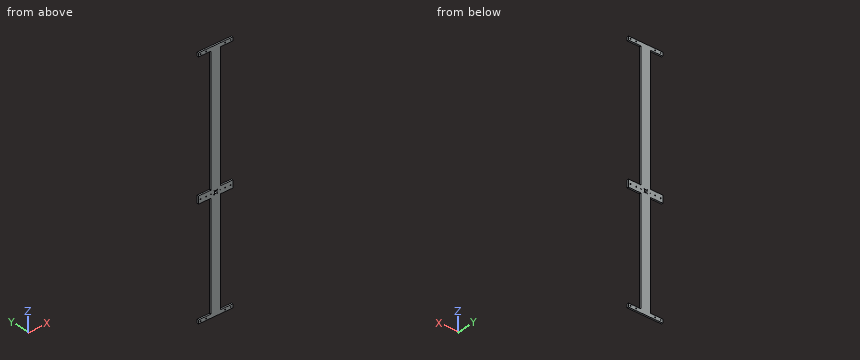
from build123d import *

# Parameters (mm, degrees)
SKETCH1_W                 = 108.8
SKETCH1_H                 = 23
MOUNT_BASE_DEPTH          = 5
SKETCH2_R                 = 1
SKETCH2_R_2               = 4.5
BRACKET_SCREW_HOLES_DEPTH = 5
SKETCH3_R                 = 1.5875
ANTENNA_SCREW_HOLES_DEPTH = 5
SKETCH6_W                 = 30
SKETCH6_H                 = 5
DIRECTOR_EXTENSION_DEPTH  = 328.35
SKETCH7_W                 = 108.8
SKETCH7_H                 = 5
DIRECTOR_MOUNT_DEPTH      = 11.5
SKETCH10_W                = 30
SKETCH10_H                = 5
REFLECTOR_EXTENSION_DEPTH = 394.02
SKETCH11_W                = 108.8
SKETCH11_H                = 5
REFLECTOR_MOUNT_DEPTH     = 11.5
LPATTERN1_COUNT           = 2
LPATTERN1_PITCH           = 411.27
LPATTERN1_COL_COUNT       = 2
LPATTERN1_COL_PITCH       = 345.6


with BuildPart() as part:
    # Sketch1 → Mount Base (new body)
    with BuildSketch(Plane(origin=(0, 0, 0), x_dir=(1, 0, 0), z_dir=(0, 1, 0))):
        with Locations((54.4, 11.5)):
            Rectangle(SKETCH1_W, SKETCH1_H)
    extrude(amount=MOUNT_BASE_DEPTH)

    # Sketch2 → Bracket Screw Holes (cut)
    with BuildSketch(Plane(origin=(0, 5, 0), x_dir=(1, 0, 0), z_dir=(0, 1, 0))):
        with Locations(Location((59.55, 16.6, 0), (0, 0, 270))):
            Circle(SKETCH2_R)
        with Locations(Location((59.55, 6.4, 0), (0, 0, 270))):
            Circle(SKETCH2_R)
        with Locations(Location((49.25, 6.4, 0), (0, 0, 270))):
            Circle(SKETCH2_R)
        with Locations(Location((49.25, 16.6, 0), (0, 0, 270))):
            Circle(SKETCH2_R)
        with Locations(Location((69.31, 11.5, 0), (0, 0, 270))):
            Circle(SKETCH2_R)
        with Locations(Location((39.49, 11.5, 0), (0, 0, 270))):
            Circle(SKETCH2_R)
        with Locations(Location((54.4, 11.5, 0), (0, 0, 270))):
            Circle(SKETCH2_R_2)
    extrude(amount=-BRACKET_SCREW_HOLES_DEPTH, mode=Mode.SUBTRACT)

    # Sketch3 → Antenna Screw Holes (cut)
    with BuildSketch(Plane(origin=(0, 5, 0), x_dir=(1, 0, 0), z_dir=(0, 1, 0))):
        with Locations(Location((6.7, 11.5, 0), (0, 0, 270))):
            Circle(SKETCH3_R)
        with Locations(Location((24.4, 11.5, 0), (0, 0, 270))):
            Circle(SKETCH3_R)
        with Locations(Location((84.4, 11.5, 0), (0, 0, 270))):
            Circle(SKETCH3_R)
        with Locations(Location((102.1, 11.5, 0), (0, 0, 270))):
            Circle(SKETCH3_R)
    antenna_screw_holes = extrude(amount=-ANTENNA_SCREW_HOLES_DEPTH, mode=Mode.SUBTRACT)

    # Sketch6 → Director Extension (add)
    with BuildSketch(Plane(origin=(0, 0, -23), x_dir=(-1, 0, 0), z_dir=(0, 0, -1))):
        with Locations((-54.4, 2.5)):
            Rectangle(SKETCH6_W, SKETCH6_H)
    extrude(amount=DIRECTOR_EXTENSION_DEPTH)

    # Sketch7 → Director Mount (add)
    with BuildSketch(Plane(origin=(0, 0, -351.35), x_dir=(-1, 0, 0), z_dir=(0, 0, -1))):
        with Locations((-54.4, 2.5)):
            Rectangle(SKETCH7_W, SKETCH7_H)
    extrude(amount=DIRECTOR_MOUNT_DEPTH)

    # Sketch10 → Reflector Extension (add)
    with BuildSketch(Plane.XY):
        with Locations((54.4, 2.5)):
            Rectangle(SKETCH10_W, SKETCH10_H)
    extrude(amount=REFLECTOR_EXTENSION_DEPTH)

    # Sketch11 → Reflector Mount (add)
    with BuildSketch(Plane.XY.offset(394.02)):
        with Locations((54.4, 2.5)):
            Rectangle(SKETCH11_W, SKETCH11_H)
    extrude(amount=REFLECTOR_MOUNT_DEPTH)

    # LPattern1: Antenna Screw Holes ×2
    with Locations(*[(0, 0, i * LPATTERN1_PITCH) for i in range(1, LPATTERN1_COUNT)]):
        add(antenna_screw_holes, mode=Mode.SUBTRACT)

    # LPattern1 col: Antenna Screw Holes ×2
    with Locations(*[(0, 0, -i * LPATTERN1_COL_PITCH) for i in range(1, LPATTERN1_COL_COUNT)]):
        add(antenna_screw_holes, mode=Mode.SUBTRACT)


solid = part.part
Could you check a few things on this model? Use its own coordinates, in mm. Round coordinates to 2 decimals unless told otherwise and drop trailing zeros. Order: outer loops, then holes, each group sorted by start corner. A loop starts at its lowest first (then second) coordinate and runs counter-clockwise, first axis right, second up.
Q1. Imagine slicing it at B-B, the plane y = 1.8. State how many separate pieces and enclosed holes the cut face has, then the cut area to 3 significant figures.
Geometry says:
separate pieces: 1
enclosed holes: 19
area: 26,500 mm2
Q2. I'm going to push flat-ended pins straight in: P1, Ø2.5, axis at y = 3.5, z = 290.5, coming from the +X side; P2, Ø1, axis at y = 1, z = -86, coming from the -X side. Where does each tip first touch, or does it pass through?
Geometry says:
P1: stops at x = 69.4
P2: stops at x = 39.4
Q3. Please list where these lines run through material, in increasing order: probe 1 along Z at (x, y) = (84.4, 1.9); probe 2 along Z at (x, y) = (97, 2.8); probe 3 along X at (y, z) = (2.8, -16.6).
Geometry says:
probe 1: z = -362.85 to -358.69, -355.51 to -351.35, -23 to -13.09, -9.91 to 0, 394.02 to 398.18, 401.36 to 405.52
probe 2: z = -362.85 to -351.35, -23 to 0, 394.02 to 405.52
probe 3: x = 0 to 48.25, 50.25 to 58.55, 60.55 to 108.8
Q4. Imagine slicing it at A-A, the plane z = -156.5. List the corners of the cut face in (x, y) for me, then the cut area to 3 significant figures.
Geometry says:
outline: (39.4, 0) - (69.4, 0) - (69.4, 5) - (39.4, 5) - close
area: 150 mm2
